Study the drawing (mm; zero at the part's minimum x, y, z) and answer. A direction names the side the tool comes from. Round coordinates to 2 decimals unless told otherwise and drop trailing zeros. Write each loop counter-clockwise with the first axis right and the second up, starting at its lowest first coordinate (ties: lowest second). Pieces come first, ordered by that corner, then holes. Notation, with made-up numbers: M 79,83 L 117,83 A10 cw 117,101 Z; hole C 72.5,88 d4. An arc over 180 degrees is marked long. Write each question's results on one line, items separated by ' | '.
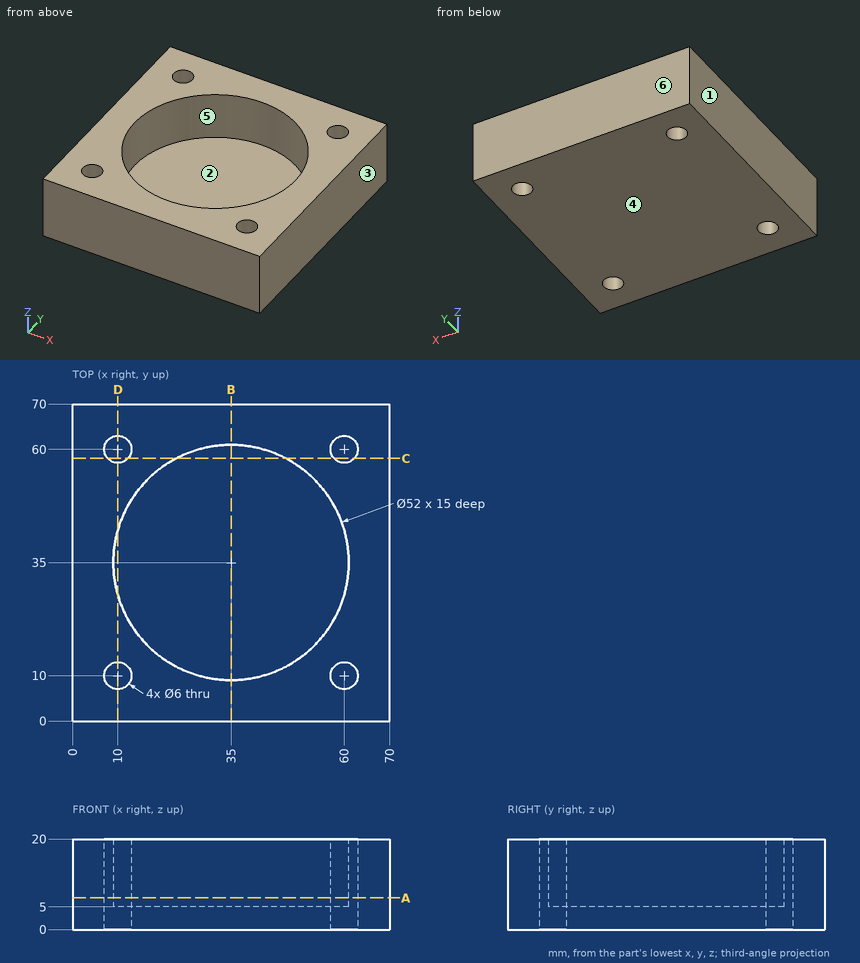
1) The mould has two halves that part along X. Classify the marked faces 1, 2, 3 and 4: +X half, -X half, draft (parallel to the pull), parting line (faces both ways), or undercut.
Return value:
face 1: -X half | face 2: undercut | face 3: +X half | face 4: draft
2) Find the intervals of material crossed by line 1 (Z direction, x = 50.5, y = 25.5); line 2 (Y direction, x = 35, z = 17.5); line 3 (X direction, y = 51, z = 16.5), in increasing order.
Return value:
line 1: 0 to 5 | line 2: 0 to 9, 61 to 70 | line 3: 0 to 14.51, 55.49 to 70
3) Section A-A (z = 7) is taken. Determine the outline of the cut face in (x, y).
Return value:
outline: M 0,0 L 70,0 L 70,70 L 0,70 Z; hole C 10,10 d6; hole C 10,60 d6; hole C 35,35 d52; hole C 60,10 d6; hole C 60,60 d6
4) Section B-B (x = 35) is taken. Determine the outline of the cut face in (y, z), then the cut area to 3 significant figures.
Return value:
outline: M 0,0 L 70,0 L 70,20 L 61,20 L 61,5 L 9,5 L 9,20 L 0,20 Z | area: 620 mm²
5) Section C-C (y = 58) is taken. Determine the outline of the cut face in (x, z), then the cut area to 3 significant figures.
Return value:
outline: M 0,0 L 7.76,0 L 7.76,20 L 0,20 Z; M 12.24,0 L 57.76,0 L 57.76,20 L 47.12,20 L 47.12,5 L 22.88,5 L 22.88,20 L 12.24,20 Z; M 62.24,0 L 70,0 L 70,20 L 62.24,20 Z | area: 857 mm²
6) Each of these flat-tipped pins is pushed along its axis until it touches: pin 1 (3 mm diameter, centred on x = 31.5, y = 20, fed in from +Z); pin 2 (3.5 mm diameter, centred on x = 60, y = 10, fed in from -Z). Where does it stop, or does it pass through?
Return value:
pin 1: z = 5 | pin 2: through
7) A tool of negligible diameter and unlimited length cuts with its end or side. For the marked faces 5 and 6, from which of +Z, -Z, +X, -X, +Y, -Y can it reach the whole face along a straight path? Write none if from no direction.
Return value:
face 5: +Z | face 6: +Z, -Z, +X, -X, +Y
8) Section D-D (x = 10) is taken. Determine the outline of the cut face in (y, z).
Return value:
outline: M 0,0 L 7,0 L 7,20 L 0,20 Z; M 13,0 L 57,0 L 57,20 L 42.14,20 L 42.14,5 L 27.86,5 L 27.86,20 L 13,20 Z; M 63,0 L 70,0 L 70,20 L 63,20 Z
